```python
from build123d import *

# Parameters (mm, degrees)
F0_W     = 32.0802
F0_H     = 238.125
F1_DEPTH = 16.0401
F3_DEPTH = 32.0802


# Not quite as in the source:
# - a pattern or mirror of a feature is missing from the dataset's text; its kind, count and spacing are read off the source's solid


with BuildPart() as f1:
    # F0 (on Top) → F1 (new body, symmetric)
    with BuildSketch(Plane.XY):
        Rectangle(F0_W, F0_H)
    extrude(amount=F1_DEPTH, both=True)

    # F2 (on face) → F3 (cut, through all)
    with BuildSketch(Plane.XY.offset(16.0401)):
        Polygon((-16.0401, -119.0625), (16.0401, -119.0625), (16.0401, -86.9823), align=None)
    f3 = extrude(amount=-F3_DEPTH, mode=Mode.SUBTRACT)

    # F3_copies: F3 across plane
    add(f3.mirror(Plane.ZX), mode=Mode.SUBTRACT)


solid = f1.part
```
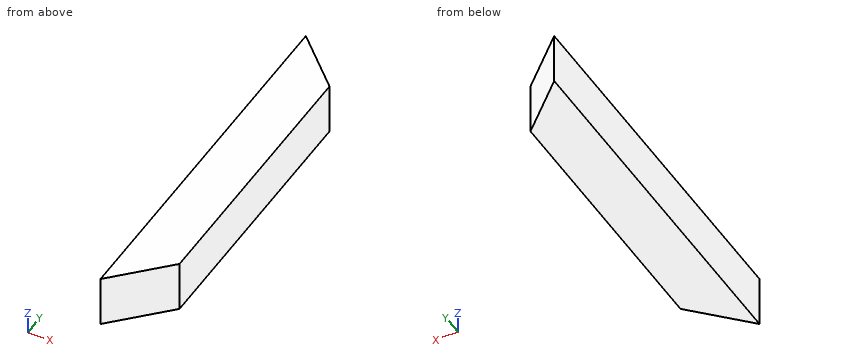
Check sheet for the modelled part. Datum: model origin and axes. Units: mm. Coordinates: 2 decimals unless noted, no trailing zeros. Loops run counter-clockwise (first coordinate to the right, second up) from the corner with the lowest first, then second, coordinate; pieces in that order, holes last.
1) Gauge pin test, flat ends, axial feed: pin 1 (12 mm diameter, centred on x = 4.5, z = 1, fed in from +Y); pin 2 (12 mm diameter, centred on x = -6, z = -3.5, fed in from -Y); pin 3 (4 mm diameter, centred on x = -10, z = -3.5, fed in from +Y). Record the tip position at first contact, or that the pin passes through.
2) Sectioned sample at B-B (x = 10). Record the boundary of the cut face in (y, z).
3) Sectioned sample at A-A (z = -1). Record the boundary of the cut face in (x, y).
4) Material ranges on probe 1 along Y at (x, z) = (0, 10.5); probe 2 along Y at (x, z) = (-5.5, 7); probe 3 along X at (y, z) = (109, -3.5), recorded low to high.
Check sheet entries:
1. pin 1: stops at y = 104.52
1. pin 2: stops at y = -115.02
1. pin 3: stops at y = 115.02
2. outline: (-93.02, -16.04) - (93.02, -16.04) - (93.02, 16.04) - (-93.02, 16.04) - close
3. outline: (-16.04, -119.06) - (16.04, -86.98) - (16.04, 86.98) - (-16.04, 119.06) - close
4. probe 1: y = -103.02 to 103.02
4. probe 2: y = -108.52 to 108.52
4. probe 3: x = -16.04 to -5.98
